Verification items for the finished model (mm, model axes). A direction names the side the tool comes from. Give positions to 0.01 mm unless a question says otherwise; leave off trailing zeros. Write each loop counter-clockwise with the first axis right and the second up, starting at its lowest first coordinate (ties: lowest second). Pieces come first, ordered by that corner, then holes. Notation, with made-up numbers: (31.25, 45.5) - (82.25, 45.5) arc R24 cw to (82.25, 65.5) - close; hole circle Ø3 at (57, -18). An arc over 180 degrees is marked (long way). Answer as a JSON object with one key per item and string values. Group by question number.
Item 1: Sectioned sample at C-C, the plane y = -9. Record the boundary of the cut face in (x, z).
Item 2: Tool access check on faces 1 (the face through (18, 35, 2)), 2 (the face through (-26, 20, 3)), 3 (the face through (-17, -34, 2.5)), 4 (the face through (-16, -30.3, 1)), 5 (the face through (22.5, 0, 3)). Record the directions out of +Z, -Z, +X, -X, +Y, -Y that give a thin tool (end or side, any length) a straight path to the whole face; none if there is none.
Item 3: Sectioned sample at D-D, the plane x = 14. Record the boundary of the cut face in (y, z), and give its area (3 significant figures).
Item 4: Go/stop test with flat-tipped pins: pin 1 (1.5 mm diameter, centred on y = -4.5, z = 2, fed in from +X); pin 2 (1.5 mm diameter, centred on x = -14.5, z = 3.5, fed in from -Y); pin 3 (1 mm diameter, centred on x = 25.5, z = 1.5, fed in from +Y). Record where each tip stops, or that it passes through.
Item 5: Sectioned sample at A-A, the plane x = -17. Record the boundary of the cut face in (y, z), and give its area (4 significant figures).
Item 6: Scan lines: line 1 along Y through (x, z) = (-25, 3.4); line 2 along Y through (x, z) = (-15.5, 2.25); line 3 along Y through (x, z) = (21.5, 3.9). Record each from-to range of solid material in increasing order. Write a range as [from, to].
Item 7: Draft check along X on faces 6 (the face through (-22.5, -33, 4)), 7 (the face through (27.5, 28, 2)), 8 (the face through (26, -20, 3)). Enter one of: +X half, -X half, draft (parallel to the pull), parting line (faces both ways), or undercut.
```python
from build123d import *

# Parameters (mm, degrees)
BOSS_EXTRUDE2_DEPTH = 5
SKETCH3_W           = 5
SKETCH3_H           = 40
CUT_EXTRUDE1_DEPTH  = 5
SKETCH5_W           = 12
SKETCH5_H           = 5
CUT_EXTRUDE2_DEPTH  = 2.5
CUT_EXTRUDE3_DEPTH  = 3.5
SKETCH7_R           = 1.5875
CUT_EXTRUDE4_DEPTH  = 6


with BuildPart() as part:
    # Sketch2 → Boss-Extrude2 (new body)
    with BuildSketch(Plane.XY):
        Polygon((-7.5, 40), (7.5, 40), (7.5, 35), (27.5, 35), (27.5, -35), (7.5, -35), (7.5, -40), (-7.5, -40), (-7.5, -35), (-27.5, -35), (-27.5, 35), (-7.5, 35), align=None)
    extrude(amount=BOSS_EXTRUDE2_DEPTH)

    # Sketch3 → Cut-Extrude1 (cut)
    with BuildSketch(Plane.XY.offset(5)):
        with Locations((-25, 0)):
            Rectangle(SKETCH3_W, SKETCH3_H)
    cut_extrude1 = extrude(amount=-CUT_EXTRUDE1_DEPTH, mode=Mode.SUBTRACT)

    # Mirror1: Cut-Extrude1 across plane
    add(cut_extrude1.mirror(Plane(origin=(0, 0, 0), x_dir=(0, 0, 1), z_dir=(1, 0, 0))), mode=Mode.SUBTRACT)

    # Sketch5 → Cut-Extrude2 (cut)
    with BuildSketch(Plane.XY.offset(5)):
        with Locations((-16.5, -32.5)):
            Rectangle(SKETCH5_W, SKETCH5_H)
    extrude(amount=-CUT_EXTRUDE2_DEPTH, mode=Mode.SUBTRACT)

    # Sketch6 → Cut-Extrude3 (cut, through all)
    with BuildSketch(Plane.XY.offset(2.5)):
        with BuildLine():
            Line((-19.72, -33.5), (-13.28, -33.5))
            ThreePointArc((-13.28, -33.5), (-12.37490332, -33.12509668), (-12, -32.22))
            Line((-12, -32.22), (-12, -31.58))
            ThreePointArc((-12, -31.58), (-12.37490332, -30.67490332), (-13.28, -30.3))
            Line((-13.28, -30.3), (-19.72, -30.3))
            ThreePointArc((-19.72, -30.3), (-20.62509668, -30.67490332), (-21, -31.58))
            Line((-21, -31.58), (-21, -32.22))
            ThreePointArc((-21, -32.22), (-20.62509668, -33.12509668), (-19.72, -33.5))
        make_face()
    extrude(amount=-CUT_EXTRUDE3_DEPTH, mode=Mode.SUBTRACT)

    # Sketch7 → Cut-Extrude4 (cut, through all)
    with BuildSketch(Plane.XY.offset(5)):
        with Locations((-7.5, 35)):
            Circle(SKETCH7_R)
        with Locations((7.5, 35)):
            Circle(SKETCH7_R)
        with Locations((22.5, 20)):
            Circle(SKETCH7_R)
        with Locations((-22.5, 20)):
            Circle(SKETCH7_R)
        with Locations((-22.5, -20)):
            Circle(SKETCH7_R)
        with Locations((-7.5, -35)):
            Circle(SKETCH7_R)
        with Locations((7.5, -35)):
            Circle(SKETCH7_R)
        with Locations((22.5, -20)):
            Circle(SKETCH7_R)
    extrude(amount=-CUT_EXTRUDE4_DEPTH, mode=Mode.SUBTRACT)


solid = part.part
```
Geometry check:
{
 "1": {"outline": "(-22.5, 0) - (22.5, 0) - (22.5, 5) - (-22.5, 5) - close"},
 "2": {"face 1": "+Z, -Z, +X, +Y", "face 2": "+Z, -Z, -X", "face 3": "+Z, -Y", "face 4": "+Z, -Z", "face 5": "+Z, -Z, +X"},
 "3": {"outline": "(-35, 0) - (35, 0) - (35, 5) - (-35, 5) - close", "area": "350 mm^2"},
 "4": {"pin 1": "x = 22.5", "pin 2": "y = -30", "pin 3": "y = 35"},
 "5": {"outline": "(-35, 0) - (-33.5, 0) - (-33.5, 2.5) - (-35, 2.5) - close; (-30.3, 0) - (35, 0) - (35, 5) - (-30, 5) - (-30, 2.5) - (-30.3, 2.5) - close", "area": "329.5 mm^2"},
 "6": {"line 1": "[-35, -20], [20, 35]", "line 2": "[-35, -33.5], [-30.3, 35]", "line 3": "[-35, -21.23], [-18.77, 18.77], [21.23, 35]"},
 "7": {"face 6": "undercut", "face 7": "+X half", "face 8": "draft"}
}
